Could you check a few things on this drawing? It's one solid part, dimensions in mm from its lowest x, y, z. A direction names the side the tool comes from. Give positions to 0.01 mm unless a question says otherwise; leave off trailing zeros. Write each loop counter-clockwise with the first axis right and the second up, starting at its lowest first coordinate (ties: lowest second). Pieces come first, ordered by that corner, then holes. Notation, with made-up numbers: M -33.75,50 L 23.25,50 A10 ccw 23.25,65 Z; hole C 54.25,13 d3. An arc over 180 degrees is marked long. Write each question's results on one line, items separated by ' | '. Start each with the question number.
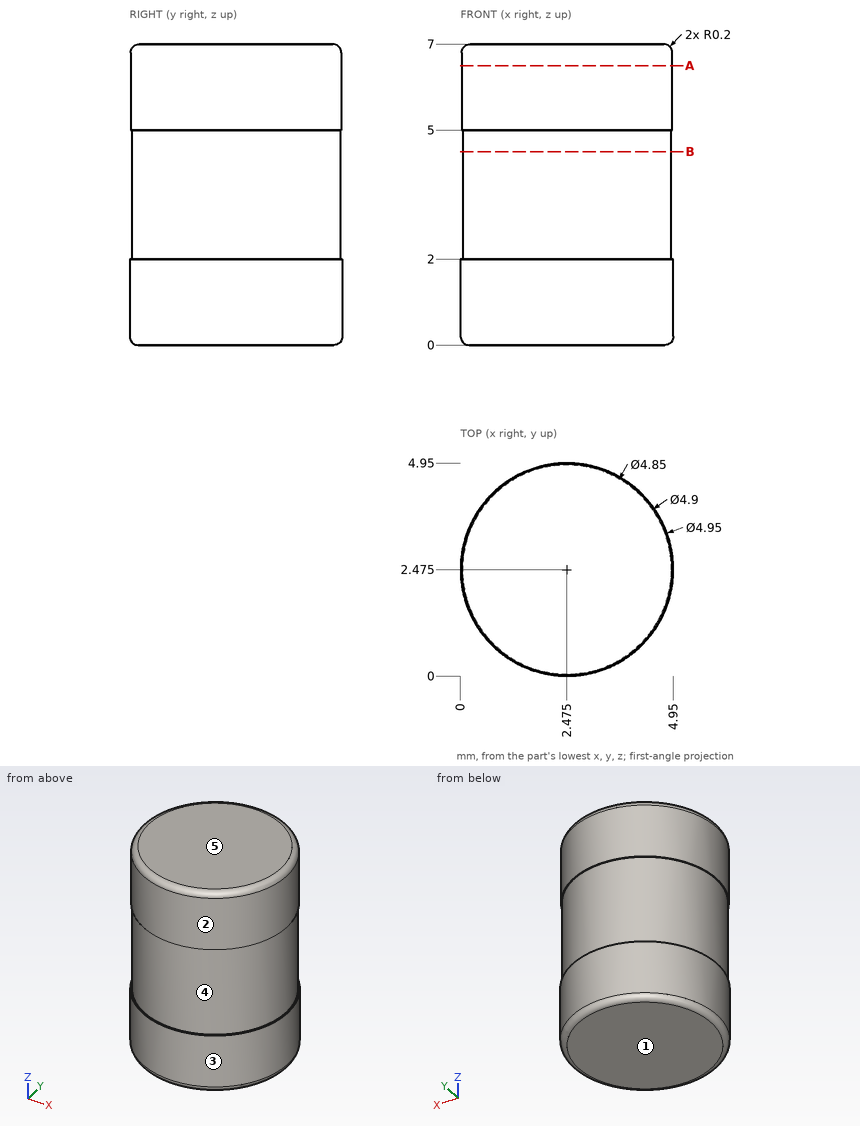
Q1. If we mould it in two halves opening along Z, with no side actions, what happens to the marked faces 3, 4 and 5? For each: pulls with the +Z half, pulls with the -Z half, needs draft (parallel to the pull), parting line crosses it, or undercut.
Q2. Please list where these lines run through material, in increasing order: line 1 (Y direction, x = 0.8, z = 5.5); line 2 (X direction, y = 1.5, z = 6.25); line 3 (X direction, y = 0.9, z = 1). Write a range as [from, to].
Q3. If we section it at B-B (z = 4.5): Please give me the cut outline in (x, y) (3 decimals), plus the area to 3 significant figures.
Q4. For the marked faces 1 and 2, which set-ups out of +Z, -Z, +X, -X, +Y, -Y let a thin tool reach every point of the face, with its end or its side?
Q5. If we section it at A-A (z = 6.5): Please give me the cut outline in (x, y) (3 decimals), plus the area to 3 significant figures.
Determined:
1) face 3: needs draft | face 4: undercut | face 5: pulls with the +Z half
2) line 1: y = [0.69, 4.26] | line 2: x = [0.23, 4.72] | line 3: x = [0.57, 4.38]
3) outline: C 2.475,2.475 d4.85 | area: 18.5 mm²
4) face 1: -Z, +X, -X, +Y, -Y | face 2: +Z
5) outline: C 2.475,2.475 d4.9 | area: 18.9 mm²
